from build123d import *

# Parameters (mm, degrees)
SKETCH2_R               = 17.78
CUT_EXTRUDE1_DEPTH      = 51.816
SKETCH3_R               = 6.35
CUT_EXTRUDE2_DEPTH      = 23.225
CUT_EXTRUDE2_DEPTH_BACK = 23.225
CUT_EXTRUDE3_START      = 19.177
SKETCH4_W               = 22.225
SKETCH4_H               = 19.05
CUT_EXTRUDE3_DEPTH      = 4.0480001
CUT_EXTRUDE4_DEPTH      = 23.225


with BuildPart() as part:
    # Sketch1 → Revolve1 (revolve)
    with BuildSketch(Plane.XY):
        with BuildLine():
            Line((0, 0), (0, 58.166))
            ThreePointArc((0, 58.166), (6.387986381, 58.484288237), (12.712693656, 59.436))
            Line((12.712693656, 59.436), (22.225, 59.436))
            Line((22.225, 59.436), (22.225, 51.816))
            Line((22.225, 51.816), (19.685, 51.816))
            Line((19.685, 51.816), (19.685, 49.276))
            Line((19.685, 49.276), (22.225, 49.276))
            Line((22.225, 49.276), (22.225, 46.736))
            Line((22.225, 46.736), (19.685, 46.736))
            Line((19.685, 46.736), (19.685, 44.196))
            Line((19.685, 44.196), (22.225, 44.196))
            Line((22.225, 44.196), (22.225, 0))
            Line((22.225, 0), (0, 0))
        make_face()
    revolve(axis=Axis((0, 0, 0), (0, 1, 0)))

    # Sketch2 → Cut-Extrude1 (cut)
    with BuildSketch(Plane.XZ):
        Circle(SKETCH2_R)
    extrude(amount=-CUT_EXTRUDE1_DEPTH, mode=Mode.SUBTRACT)

    # Sketch3 → Cut-Extrude2 (cut, two sides)
    with BuildSketch(Plane.XY) as cut_extrude2_sk:
        with Locations((0, 30.48)):
            Circle(SKETCH3_R)
    extrude(amount=CUT_EXTRUDE2_DEPTH, mode=Mode.SUBTRACT)
    extrude(cut_extrude2_sk.sketch, amount=-CUT_EXTRUDE2_DEPTH_BACK, mode=Mode.SUBTRACT)

    # Sketch4 → Cut-Extrude3 (cut, through all)
    with BuildSketch(Plane.XY.offset(CUT_EXTRUDE3_START)):
        with Locations((0.0635, 30.48)):
            Rectangle(SKETCH4_W, SKETCH4_H)
    cut_extrude3 = extrude(amount=CUT_EXTRUDE3_DEPTH, mode=Mode.SUBTRACT)

    # Mirror1: Cut-Extrude3 across plane
    add(cut_extrude3.mirror(Plane.XY), mode=Mode.SUBTRACT)

    # Sketch5 → Cut-Extrude4 (cut, symmetric)
    with BuildSketch(Plane.XY):
        with BuildLine():
            Line((22.225, 0), (22.225, 7.62))
            Line((22.225, 7.62), (13.343533586, 7.62))
            ThreePointArc((13.343533586, 7.62), (11.546046061, 7.169336035), (10.173788381, 5.923957269))
            Line((10.173788381, 5.923957269), (6.223, 0))
            Line((6.223, 0), (22.225, 0))
        make_face()
    cut_extrude4 = extrude(amount=CUT_EXTRUDE4_DEPTH, both=True, mode=Mode.SUBTRACT)

    # Mirror2: Cut-Extrude4 across plane
    add(cut_extrude4.mirror(Plane(origin=(0, 0, 0), x_dir=(0, 0, 1), z_dir=(1, 0, 0))), mode=Mode.SUBTRACT)


solid = part.part
Source: CAD feature listing. Evaluate the final solid. Frame: model axes, mm. A direction names the side the tool comes from. Give positions to 0.01 mm unless a question says otherwise; leave off trailing zeros. Write each loop counter-clockwise with the first axis right and the second up, starting at its lowest first coordinate (ties: lowest second). Pieces come first, ordered by that corner, then holes. Notation, with made-up numbers: M 44,25.5 L 75,25.5 A23 cw 75,35.5 Z; hole C 36.25,-25 d10. An arc over 180 degrees is marked long. Answer as a JSON object with one key per item and string values.
Q1. Access query for faces 4 (the face through (0, 51.816, 0)), 5 (the face through (-18, 7.62, 0)). Directions: +Z, -Z, +X, -X, +Y, -Y. A direction counts if a zero-diameter tool reaches every point of the face in a straight line with its end or side. Return the directions, or none.
Geometry check:
{"face 4": "-Y", "face 5": "+Z, -Z, -X, -Y"}
Q2. Ray query, line 1 along Z through (x, y) = (-0.5, 24); line 2 along X through (y, z) = (26, 0) (3 decimals); line 3 along Y through (x, z) = (-16, 14.5). Return the intervals inside material, ascending.
Geometry check:
{"line 1": "z = -19.18 to -17.77, 17.77 to 19.18", "line 2": "x = -22.225 to -17.78, 17.78 to 22.225", "line 3": "y = 7.62 to 44.2, 46.74 to 49.28, 51.82 to 59.44"}
Q3. Cut plane C-C, the plane z = 0. Return the cut outline in (x, y) (3 decimals).
Geometry check:
{"outline": "M -22.225,7.62 L -17.78,7.62 L -17.78,51.816 L 17.78,51.816 L 17.78,7.62 L 22.225,7.62 L 22.225,44.196 L 19.685,44.196 L 19.685,46.736 L 22.225,46.736 L 22.225,49.276 L 19.685,49.276 L 19.685,51.816 L 22.225,51.816 L 22.225,59.436 L 12.713,59.436 A64.262 cw -12.713,59.436 L -22.225,59.436 L -22.225,51.816 L -19.685,51.816 L -19.685,49.276 L -22.225,49.276 L -22.225,46.736 L -19.685,46.736 L -19.685,44.196 L -22.225,44.196 Z"}
Q4. Cut plane A-A, the plane y = 30.48. Return the cut outline in (x, z) (3 decimals).
Geometry check:
{"outline": "M -11.049,-19.284 L -11.049,-19.177 L -6.35,-19.177 L -6.35,-16.607 A17.78 cw -6.35,16.607 L -6.35,19.177 L -11.049,19.177 L -11.049,19.284 A22.225 ccw Z; M 6.35,-19.177 L 11.176,-19.177 L 11.176,-19.211 A22.225 ccw 11.176,19.211 L 11.176,19.177 L 6.35,19.177 L 6.35,16.607 A17.78 cw 6.35,-16.607 Z"}
Q5. Cut plane D-D, the plane y = 15. Return the cut outline in (x, z) (3 decimals), then the cut area to 3 significant figures.
Geometry check:
{"outline": "C 0,0 d44.45; hole C 0,0 d35.56", "area": "559 mm^2"}
Q6. Cut plane B-B, the plane x = 0. Count the separate pieces of the cut face and the enclosed holes in it, then the cut area to 3 significant figures.
Geometry check:
{"separate pieces": "3", "enclosed holes": "0", "area": "600 mm^2"}
Q7. Contact query for flat-ended pins moving along their axis: P1, Ø0.9, axis at x = 3.5, z = -21, coming from the -Y side; P2, Ø5, axis at y = 48.5, z = -14.5, coming from the +X side; P3, Ø14.5, axis at x = 0, y = 30.48, coming from the +Z side; P4, Ø10, axis at x = 10, y = 21.5, coming from the -Z side. Output: stop coordinate, or through.
Geometry check:
{"P1": "stops at y = 0", "P2": "stops at x = 18.71", "P3": "stops at z = 19.18", "P4": "stops at z = -21.65"}
Q8. Mould query, pull axis X, two halves, no side actions, for faces 1 (the face through (16.424, 25.545, -6.81)), 2 (the face through (8.226, 3.003, 18.006)), 3 (the face through (-15.62, 50.53, 11.98)). Classes: +X half, -X half, draft (parallel to the pull), parting line (faces both ways), or undercut.
Geometry check:
{"face 1": "undercut", "face 2": "+X half", "face 3": "parting line"}
